Source: CAD feature listing. Evaluate the final solid. Frame: model axes, mm. Face numbers are marked on the shaded views. Give positions to 0.01 mm unless a question says otherwise; leave off trailing zeros. Loops run counter-clockwise (first coordinate to the right, second up) from the corner with the lowest first, then second, coordinate; pieces in that order, holes last. Notation, with made-up numbers: (10.5, -15) - (20.5, -15) arc R18 cw to (20.5, 15) - close; hole circle Ø10 at (-2, 40). An arc over 180 degrees is marked (long way). Put each result on its own line as item: value.
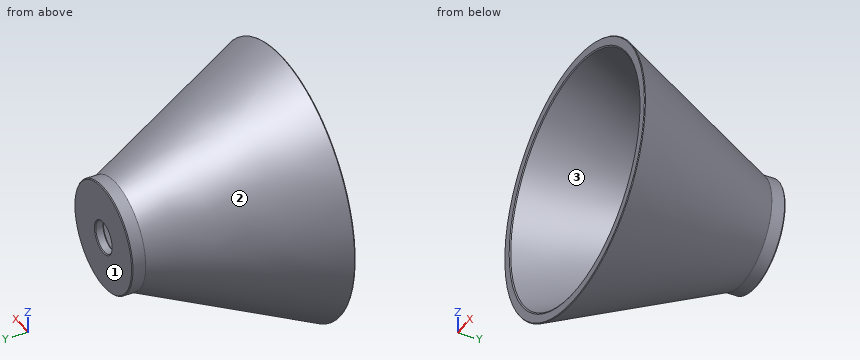
Autodesk Inventor part; units mm, degrees
ref_plane "YZ Plane" through (0, 0, 0) normal (1, 0, 0) x (0, 1, 0)
ref_plane "XZ Plane" through (0, 0, 0) normal (0, 1, 0) x (-1, 0, 0)
ref_plane "XY Plane" through (0, 0, 0) normal (0, 0, 1) x (1, 0, 0)
sketch "Sketch1" plane through (0, 0, 0) normal (0, 0, 1) x (1, 0, 0)
  line L0 (0, 0) -> (0, -20) construction
  line L1 (0, 0) -> (6, 0)
  line L2 (6, 0) -> (6, -1.5)
  line L3 (6, -1.5) -> (14.6267, -20)
  line L4 (13.5233, -20) -> (4.9604, -1.6369)
  line L5 (4.9604, -1.6369) -> (4.9604, -1)
  line L6 (4.9604, -1) -> (0, -1)
  line L7 (0, 0) -> (0, -1)
  line L8 (14.6267, -20) -> (13.5233, -20)
  dimension "d1" = 6
  dimension "d2" = 1.5
  dimension "d3" = 25
  dimension "d4" = 20
  dimension "d5" = 1
  dimension "d6" = 1
revolve "Revolution1" add sketch "Sketch1" angle 360 about axis through (0, 0, 0) along (0, -1, 0)
chamfer "Chamfer1" distance 0.1 angle 45 3 edges at (-14.6267, -20, 0) (-13.5233, -20, 0) (-6, 0, 0)
sketch "Sketch2" plane through (0, 0, 0) normal (0, 1, 0) x (1, 0, 0)
  point P0 (0, 0)
  point P1 (0, 0)
hole "Hole1" at (0, 0, 0) direction (0, -1, 0) diameter 3.5 depth 53.6 tip angle 118
chamfer "Chamfer2" distance 0.1 angle 45 2 edges at (0, 0, -1.75) (0, -1, -1.75)
properties part number "Bell" material "Brass, Soft Yellow"
1) Section query D-D, the plane y = -2.25. Output: boundary loops of the cut face in (x, z).
Check result:
outline: circle Ø12.7 at (0, 0); hole circle Ø10.49 at (0, 0)
2) Section query B-B, the plane z = 0. Output: boundary loops of the cut face in (x, y).
Check result:
outline: (-14.58, -19.91) - (-14.53, -20) - (-13.62, -20) - (-13.48, -19.91) - (-4.96, -1.64) - (-4.96, -1) - (-1.85, -1) - (-1.75, -0.9) - (-1.75, -0.1) - (-1.85, 0) - (-5.9, 0) - (-6, -0.1) - (-6, -1.5) - close; (1.75, -0.9) - (1.85, -1) - (4.96, -1) - (4.96, -1.64) - (13.48, -19.91) - (13.62, -20) - (14.53, -20) - (14.58, -19.91) - (6, -1.5) - (6, -0.1) - (5.9, 0) - (1.85, 0) - (1.75, -0.1) - close
3) Section query A-A, the plane x = 0. Output: boundary loops of the cut face in (y, z).
Check result:
outline: (-20, -14.53) - (-19.91, -14.58) - (-1.5, -6) - (-0.1, -6) - (0, -5.9) - (0, -1.85) - (-0.1, -1.75) - (-0.9, -1.75) - (-1, -1.85) - (-1, -4.96) - (-1.64, -4.96) - (-19.91, -13.48) - (-20, -13.62) - close; (-20, 13.62) - (-19.91, 13.48) - (-1.64, 4.96) - (-1, 4.96) - (-1, 1.85) - (-0.9, 1.75) - (-0.1, 1.75) - (0, 1.85) - (0, 5.9) - (-0.1, 6) - (-1.5, 6) - (-19.91, 14.58) - (-20, 14.53) - close
4) Material intervals for line 1 along Z through (x, y) = (0, -1.4); line 2 along Z through (x, y) = (0, -0.4); line 3 along Y through (x, z) = (-1.75, -4.25), sorted ascending. Write a range as [from, to].
Check result:
line 1: [-6, -4.96], [4.96, 6]
line 2: [-6, -1.75], [1.75, 6]
line 3: [-1, 0]
5) Mould query, pull axis X, two halves, no side actions, for the marked faces 1, 2 and 3. Classes: pulls with the +X half, pulls with the -X half, needs draft (parallel to the pull), parting line crosses it, or undercut.
Check result:
face 1: needs draft
face 2: parting line crosses it
face 3: undercut
6) Section query C-C, the plane y = -10.5. Output: boundary loops of the cut face in (x, z).
Check result:
outline: circle Ø20.39 at (0, 0); hole circle Ø18.19 at (0, 0)
7) Pin query (flat end, axial travel): P1, Ø4.5, axis at x = 0, z = 0, coming from the +Y side; P2, Ø8, axis at x = -1.5, z = -0.5, coming from the -Y side; P3, Ø5, axis at x = 11.5, y = -16.5, coming from the -Z side; P4, Ø8, axis at x = 0, z = 0, coming from the -Y side. Return the tip coordinate at first contact, or that it passes through.
Check result:
P1: y = 0
P2: y = -2.97
P3: z = -9.87
P4: y = -1
